Verification items for the finished model (mm, model axes). Face numbers are marked on the shaded views. A direction names the side the tool comes from. Coordinates: 2 decimals unless noted, no trailing zeros. Write each loop counter-clockwise with the first axis right and the second up, starting at its lowest first coordinate (ties: lowest second). Pieces come first, ordered by that corner, then holes. Notation, with made-up numbers: M -15.5,10.25 L -2.5,10.25 A25 ccw -2.5,30.25 Z; hole C 85,17 d10. An arc over 180 degrees is marked long. Answer in a Markdown table with one row per item.
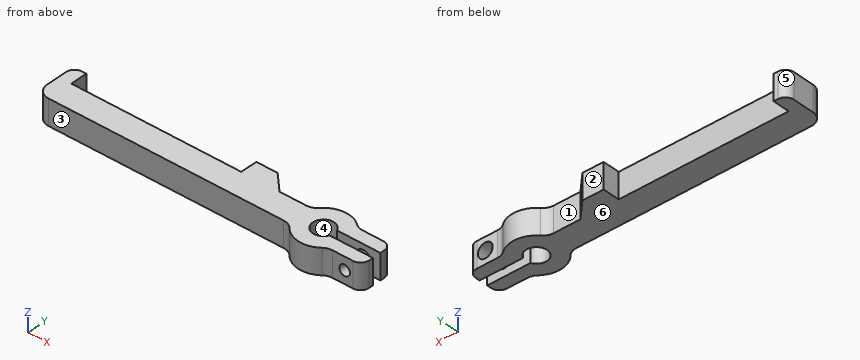
from build123d import *

# Parameters (mm, degrees)
ESQUISSE1_R                  = 6
ESQUISSE1_R_2                = 2.5
BOSS_EXTRU_1_DEPTH           = 6
ESQUISSE2_W                  = 62
ESQUISSE2_H                  = 6
BOSS_EXTRU_2_DEPTH           = 6
ESQUISSE3_W                  = 10
ESQUISSE3_H                  = 8
BOSS_EXTRU_3_DEPTH           = 6
CONG_1_R                     = 3
ENL_V_MAT_EXTRU_1_DEPTH      = 66.551506466
ENL_V_MAT_EXTRU_1_DEPTH_BACK = 66.551506466
ESQUISSE4_W                  = 12
ESQUISSE4_H                  = 2
ENL_V_MAT_EXTRU_2_DEPTH      = 67.037867924
ENL_V_MAT_EXTRU_2_DEPTH_BACK = 67.037867924
ESQUISSE5_R                  = 1.25
ESQUISSE6_R                  = 1.75
ENL_V_MAT_EXTRU_3_DEPTH      = 3
CONG_2_R                     = 2
ESQUISSE7_W                  = 3
ESQUISSE7_H                  = 4
BOSS_EXTRU_4_DEPTH           = 6
CHANFREIN1_SIZE              = 6
CONG_3_R                     = 2


with BuildPart() as part:
    # Esquisse1 → Boss.-Extru.1 (new body)
    with BuildSketch(Plane.XY):
        Circle(ESQUISSE1_R)
        Circle(ESQUISSE1_R_2, mode=Mode.SUBTRACT)
    extrude(amount=BOSS_EXTRU_1_DEPTH)

    # Esquisse2 → Boss.-Extru.2 (add)
    with BuildSketch(Plane.XY.offset(6)):
        with Locations((-34, 0)):
            Rectangle(ESQUISSE2_W, ESQUISSE2_H)
    extrude(amount=-BOSS_EXTRU_2_DEPTH)

    # Esquisse3 → Boss.-Extru.3 (add)
    with BuildSketch(Plane.XY.offset(6)):
        with Locations((7.5, 0)):
            Rectangle(ESQUISSE3_W, ESQUISSE3_H)
    extrude(amount=-BOSS_EXTRU_3_DEPTH)

    # Congé1
    cong_1_edges = [part.edges().sort_by_distance(p)[0] for p in [
        (-5.196152423, -3, 3),
        (-5.196152423, 3, 3),
        (-65, -3, 3),
        (4.472135955, -4, 3),
        (4.472135955, 4, 3),
    ]]
    fillet(cong_1_edges, radius=CONG_1_R)

    # Esquisse4 → Enlèv. mat.-Extru.1 (cut, two sides: drawn at the far end of the back side and taken through both)
    with BuildSketch(Plane.XY.offset(6).offset(-ENL_V_MAT_EXTRU_1_DEPTH_BACK)):
        with Locations((6.5, 0)):
            Rectangle(ESQUISSE4_W, ESQUISSE4_H)
    extrude(amount=ENL_V_MAT_EXTRU_1_DEPTH + ENL_V_MAT_EXTRU_1_DEPTH_BACK, mode=Mode.SUBTRACT)

    # Esquisse5 → Enlèv. mat.-Extru.2 (cut, two sides: drawn at the far end of the back side and taken through both)
    with BuildSketch(Plane(origin=(0, 4, 0), x_dir=(1, 0, 0), z_dir=(0, 1, 0)).offset(-ENL_V_MAT_EXTRU_2_DEPTH_BACK)):
        with Locations(Location((8.5, -3, 0), (0, 0, 90))):
            Circle(ESQUISSE5_R)
    extrude(amount=ENL_V_MAT_EXTRU_2_DEPTH + ENL_V_MAT_EXTRU_2_DEPTH_BACK, mode=Mode.SUBTRACT)

    # Esquisse6 → Enlèv. mat.-Extru.3 (cut)
    with BuildSketch(Plane(origin=(0, 4, 0), x_dir=(1, 0, 0), z_dir=(0, 1, 0))):
        with Locations(Location((8.5, -3, 0), (0, 0, 180))):
            Circle(ESQUISSE6_R)
    extrude(amount=-ENL_V_MAT_EXTRU_3_DEPTH, mode=Mode.SUBTRACT)

    # Congé2
    cong_2_edges = [part.edges().sort_by_distance(p)[0] for p in [
        (12.5, -4, 3),
        (12.5, 4, 3),
    ]]
    fillet(cong_2_edges, radius=CONG_2_R)

    # Esquisse7 → Boss.-Extru.4 (add)
    with BuildSketch(Plane.XY.offset(6)):
        with Locations((-63.5, 5)):
            Rectangle(ESQUISSE7_W, ESQUISSE7_H)
        with Locations((-20.5, 5)):
            Rectangle(ESQUISSE7_W, ESQUISSE7_H)
    extrude(amount=-BOSS_EXTRU_4_DEPTH)

    # Chanfrein1
    # the kernel refuses this chamfer: 6 mm, written as the material it adds along each edge
    with BuildSketch(Plane(origin=(-19, 3, 6), x_dir=(-0.027495876610586202, 0.9996219169112968, 0), z_dir=(0, 0, -1))) as chanfrein1_piece_1_section:
        Polygon((CHANFREIN1_SIZE * 0.999621916911, CHANFREIN1_SIZE * 0.0274958766106), (-CHANFREIN1_SIZE * 0.0274958766106, CHANFREIN1_SIZE * 0.999621916911), (0, 0), align=None)
    chanfrein1_piece_1 = extrude(amount=6, mode=Mode.PRIVATE)
    chanfrein1_piece_1 = split(chanfrein1_piece_1, bisect_by=Plane(origin=(-16.81581799, 7, 3), z_dir=(0, -1, 0)), keep=Keep.TOP, mode=Mode.PRIVATE)
    add(chanfrein1_piece_1)

    # Congé3
    cong_3_edges = [part.edges().sort_by_distance(p)[0] for p in [
        (-65, 7, 3),
    ]]
    fillet(cong_3_edges, radius=CONG_3_R)


solid = part.part
1) Sectioned sample at D-D (x = -45). Record the cut outline in (y, z), then the cut area to 3 significant figures.
Response values:
| item | result |
|---|---|
| outline | M -3,0 L 3,0 L 3,6 L -3,6 Z |
| area | 36.0 mm² |
2) Release check for a two-part mould opening along X. For the marked faces 4, 5 and 6 record: +X half, -X half, draft (parallel to the pull), parting line (faces both ways), or undercut.
Response values:
| item | result |
|---|---|
| face 4 | undercut |
| face 5 | -X half |
| face 6 | draft |
3) Tool access check on the marked faces 1, 2 and 3. Record the directions out of +Z, -Z, +X, -X, +Y, -Y that give a thin tool (end or side, any length) a straight path to the whole face; none if there is none.
Response values:
| item | result |
|---|---|
| face 1 | +Z, -Z, +Y |
| face 2 | +Z, -Z, +X, -X, +Y |
| face 3 | +Z, -Z, -X, -Y |
4) Depth check by flat-ended pin: pin 1 (1.5 mm diameter, centred on x = 2, z = 4.5, fed in from -Y); pin 2 (3 mm diameter, centred on x = 8.5, z = 3, fed in from +Y); pin 3 (2 mm diameter, centred on x = -23.5, z = 2, fed in from -Y). Enter the tip coordinate at first touch or a pass-through.
Response values:
| item | result |
|---|---|
| pin 1 | stops at y = -5.87 |
| pin 2 | stops at y = -1 |
| pin 3 | stops at y = -3 |
5) Sectioned sample at B-B (x = 8.5). Record the cut outline in (y, z).
Response values:
| item | result |
|---|---|
| outline | M -4,0 L -1,0 L -1,1.75 L -4,1.75 Z; M -4,4.25 L -1,4.25 L -1,6 L -4,6 Z; M 1,0 L 4,0 L 4,1.25 L 1,1.25 Z; M 1,4.75 L 4,4.75 L 4,6 L 1,6 Z |
6) Thickness scan on L1, parallel to Z at x = 8.5, y = 1.7; L2, parallel to Y at x = 0, z = 3; L3, parallel to X at y = -1.55, z = 3. Record the ranges inside material, lowest first. Write a range as [from, to].
Response values:
| item | result |
|---|---|
| L1 | z = [0, 1.25], [4.75, 6] |
| L2 | y = [-6, -2.5], [2.5, 6] |
| L3 | x = [-64.57, -1.96], [1.96, 7.25], [9.75, 12.5] |
7) Sectioned sample at A-A (x = 0). Record the cut outline in (y, z), then the cut area to 3 significant figures.
Response values:
| item | result |
|---|---|
| outline | M -6,0 L -2.5,0 L -2.5,6 L -6,6 Z; M 2.5,0 L 6,0 L 6,6 L 2.5,6 Z |
| area | 42.0 mm² |
8) Sectioned sample at C-C (z = 3). Give the number of separate pieces and of enclosed holes in the cut face, then the cut area to 3 significant figures.
Response values:
| item | result |
|---|---|
| separate pieces | 3 |
| enclosed holes | 0 |
| area | 503 mm² |
